```python
from build123d import *

# Parameters (mm, degrees)
BOSS_EXTRUDE1_DEPTH = 20.75
SKETCH2_R           = 2.75
CUT_EXTRUDE1_DEPTH  = 20.75
SKETCH3_W           = 2
SKETCH3_H           = 18.75
CUT_EXTRUDE2_DEPTH  = 20.75
FILLET1_R           = 2
BOSS_EXTRUDE2_DEPTH = 2


with BuildPart() as part:
    # Sketch1 → Boss-Extrude1 (new body)
    with BuildSketch(Plane(origin=(0, 0, 0), x_dir=(1, 0, 0), z_dir=(0, 1, 0))):
        with BuildLine():
            Line((-30, 0), (0, 0))
            Line((0, 0), (30, 0))
            Line((30, 0), (30, 4))
            Line((30, 4), (27, 4))
            ThreePointArc((27, 4), (26.414213562, 2.585786438), (25, 2))
            Line((25, 2), (-25, 2))
            ThreePointArc((-25, 2), (-26.414213562, 2.585786438), (-27, 4))
            Line((-27, 4), (-30, 4))
            Line((-30, 4), (-30, 0))
        make_face()
        with BuildLine():
            Line((27, 4), (30, 4))
            Line((30, 4), (30, 8))
            Line((30, 8), (-30, 8))
            Line((-30, 8), (-30, 4))
            Line((-30, 4), (-27, 4))
            ThreePointArc((-27, 4), (-26.414213562, 5.414213562), (-25, 6))
            Line((-25, 6), (25, 6))
            ThreePointArc((25, 6), (26.414213562, 5.414213562), (27, 4))
        make_face()
    extrude(amount=BOSS_EXTRUDE1_DEPTH)

    # Sketch2 → Cut-Extrude1 (cut)
    with BuildSketch(Plane.XY):
        Polygon((-30, 20.75), (-30, 2), (-1, 2), (-1, 11.25), (-4.75, 11.25), (-4.75, 20.75), align=None)
        with Locations((0, 16)):
            Circle(SKETCH2_R)
        Polygon((4.75, 11.25), (1, 11.25), (1, 2), (30, 2), (30, 20.75), (4.75, 20.75), align=None)
    extrude(amount=-CUT_EXTRUDE1_DEPTH, mode=Mode.SUBTRACT)

    # Sketch3 → Cut-Extrude2 (cut)
    with BuildSketch(Plane(origin=(4.75, 0, 0), x_dir=(0, 0, -1), z_dir=(1, 0, 0))):
        with Locations((7, 11.375)):
            Rectangle(SKETCH3_W, SKETCH3_H)
    extrude(amount=-CUT_EXTRUDE2_DEPTH, mode=Mode.SUBTRACT)

    # Fillet1
    fillet1_edges = [part.edges().sort_by_distance(p)[0] for p in [
        (4.75, 20.75, -1),
        (-4.75, 20.75, -1),
        (30, 1, -8),
        (30, 1, 0),
        (-30, 1, 0),
        (-30, 1, -8),
        (-4.75, 11.25, -1),
        (4.75, 11.25, -1),
    ]]
    fillet(fillet1_edges, radius=FILLET1_R)

    # Sketch5 → Boss-Extrude2 (add)
    with BuildSketch(Plane(origin=(1, 0, 0), x_dir=(0, 0, -1), z_dir=(1, 0, 0))):
        Polygon((2, 11.25), (8, 2), (6, 2), (2, 8.166666667), align=None)
    extrude(amount=-BOSS_EXTRUDE2_DEPTH)


solid = part.part
```
Design review of the part built by this model. Coordinates are the model's own, in mm. A direction names the side the tool comes from. Coordinates: 2 decimals unless noted, no trailing zeros. Loops run counter-clockwise (first coordinate to the right, second up) from the corner with the lowest first, then second, coordinate; pieces in that order, holes last.
Q1. For pin 1 (2 mm diameter, centred on y = 16, z = -1, fed in from +X); pin 2 (10.5 mm diameter, centred on x = -0.5, y = 17.5, fed in from -Z); pin 3 (4 mm diameter, centred on y = 6, z = -5, fed in from +X), all flat-tipped, find the tip position at first contact; note any pin that passes through.
Reported:
pin 1: stops at x = 4.75
pin 2: stops at z = -2
pin 3: stops at x = 1
Q2. To check wall thickness, follow line 1 (Z direction, x = -9.5, y = 1.5); line 2 (Y direction, x = 0, z = -1); line 3 (Z direction, x = 3, y = 15.75). State the ranges of each line that lie inside material, in increasing order.
Reported:
line 1: z = -8 to -6, -2 to 0
line 2: y = 0 to 13.25, 18.75 to 20.75
line 3: z = -2 to 0
Q3. We need section D-D on x = 6. State the section outline as (y, z) points, and give its area (3 significant figures).
Reported:
outline: (0, -8) - (2, -8) - (2, -6) - (0, -6) - close; (0, -2) - (2, -2) - (2, 0) - (0, 0) - close
area: 8.00 mm2
Q4. We need section B-B on z = -3. State the section outline as (x, y) points (3 decimals).
Reported:
outline: (-30, 0) - (-26.732, 0) - (-26.732, 2) - (-30, 2) - close; (-1, 6.625) - (1, 6.625) - (1, 9.708) - (-1, 9.708) - close; (26.732, 0) - (30, 0) - (30, 2) - (26.732, 2) - close
Q5. Tool access review of faces 1 (the face through (2, 11.25, -1)), 2 (the face through (-4.15, 11.82, -1.01)), 3 (the face through (0, 2, -2)): name each direction out of +Z, -Z, +X, -X, +Y, -Y from which nothing blocks a thin tool from reaching the whole face with its end or side.
Reported:
face 1: +Z, -Z, +X
face 2: +Z, -Z, -X
face 3: -Y
Q6. The part is to be moulded in two halves that separate along Y. For faces 4 (the face through (0, 0, -1)), 5 (the face through (-1, 7, -3)), 6 (the face through (0.01, 6.69, -4.96)), 7 (the face through (-29.4, 1.01, -0.57)), say which applies: +Y half, -Y half, draft (parallel to the pull), parting line (faces both ways), or undercut.
Reported:
face 4: -Y half
face 5: undercut
face 6: +Y half
face 7: draft
Q7. We need section C-C on y = 16. State the section outline as (x, z) points, and give its area (3 significant figures).
Reported:
outline: (-4.75, -2) - (-2.75, -2) - (-2.75, 0) - (-4.75, 0) - close; (2.75, -2) - (4.75, -2) - (4.75, 0) - (2.75, 0) - close
area: 8.00 mm2
Q8. We need section A-A on x = 0. State the section outline as (y, z) points, and give its area (3 significant figures).
Reported:
outline: (0, -8) - (2, -8) - (11.25, -2) - (13.25, -2) - (13.25, 0) - (0, 0) - (0, -2) - (8.17, -2) - (2, -6) - (0, -6) - close; (18.75, -2) - (20.75, -2) - (20.75, 0) - (18.75, 0) - close
area: 49.9 mm2
